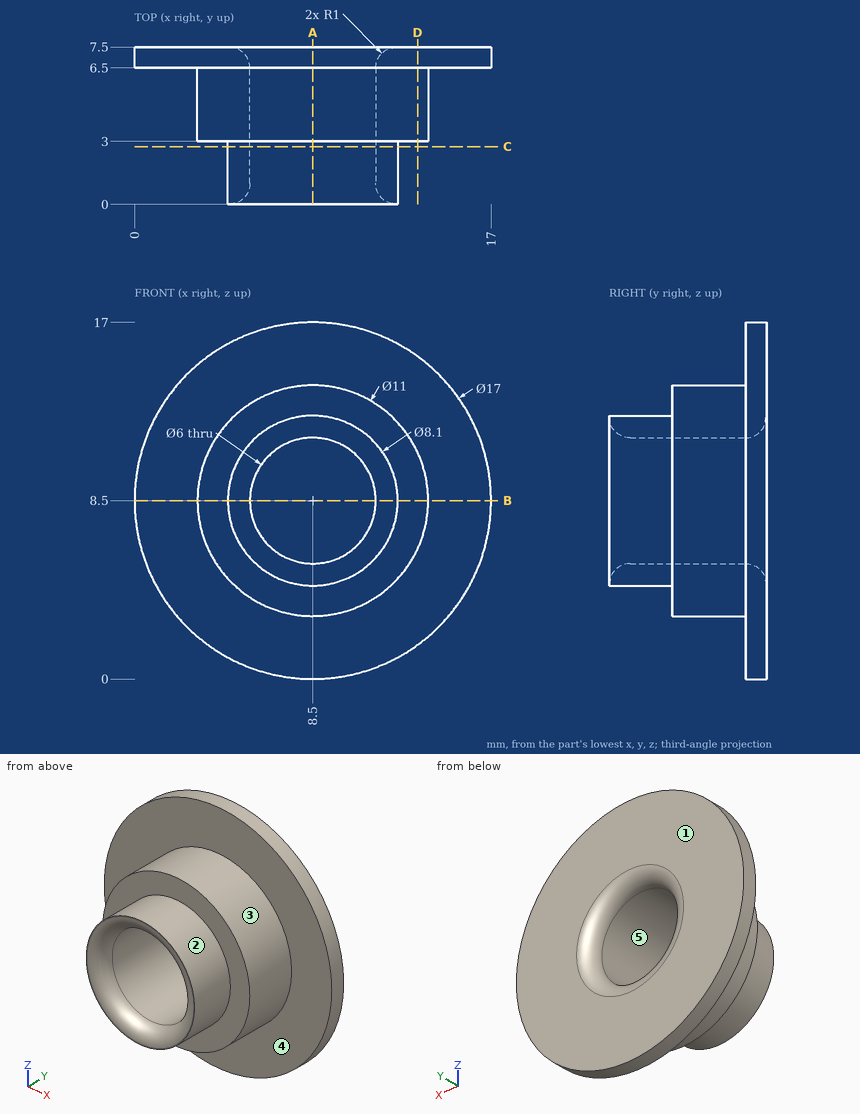
Geometry: see drawing. Coordinates: mm, zero at the bounding-box minimum. A direction names the side the tool comes from. Give positions to 0.01 mm unless a question says otherwise; leave off trailing zeros. Order: outer loops, then holes, each group sorted by start corner. A loop starts at its lowest first (then second) coordinate and runs counter-clockwise, first axis right, second up.
Q1. Section A-A on x = 8.5. Output: boundary loops of the cut face in (y, z).
Checked values:
outline: (0, 4.45) - (3, 4.45) - (3, 3) - (6.5, 3) - (6.5, 0) - (7.5, 0) - (7.5, 4.5) arc R1 ccw to (6.5, 5.5) - (1, 5.5) arc R1 ccw to (0, 4.5) - close; (0, 12.5) arc R1 ccw to (1, 11.5) - (6.5, 11.5) arc R1 ccw to (7.5, 12.5) - (7.5, 17) - (6.5, 17) - (6.5, 14) - (3, 14) - (3, 12.55) - (0, 12.55) - close
Q2. Ray query, probe 1 along Z at (x, y) = (8.5, 3.5); probe 2 along Y at (x, z) = (15.5, 8.25); probe 3 along X at (y, z) = (1, 6.25). Return the intervals inside material, ascending.
Checked values:
probe 1: z = 3 to 5.5, 11.5 to 14
probe 2: y = 6.5 to 7.5
probe 3: x = 5.13 to 6.52, 10.48 to 11.87
Q3. Section D-D on x = 13.5. Output: boundary loops of the cut face in (y, z).
Checked values:
outline: (3, 6.21) - (6.5, 6.21) - (6.5, 1.63) - (7.5, 1.63) - (7.5, 15.37) - (6.5, 15.37) - (6.5, 10.79) - (3, 10.79) - close
Q4. Section C-C on y = 2.75. Output: boundary loops of the cut face in (x, z).
Checked values:
outline: circle Ø8.1 at (8.5, 8.5); hole circle Ø6 at (8.5, 8.5)
Q5. Draft query along Z for the marked faces 3, 4 and 5. Return one class per face: +Z half, -Z half, draft (parallel to the pull), parting line (faces both ways), or undercut.
Checked values:
face 3: parting line
face 4: draft
face 5: undercut
Q6. Contact query for flat-ended pins moving along their axis: pin 1 Ø3 at (x, z) = (3.5, 3) entering from -Y; pin 2 Ø1 at (x, z) = (12, 4) entering from -Y. Output: stop coordinate, or through.
Checked values:
pin 1: stops at y = 6.5
pin 2: stops at y = 3
Q7. Set-up query: the marked faces 1 and 2. Return all of +Z, -Z, +X, -X, +Y, -Y with unobstructed straight access to the full face (end or side cutting, diameter ignored); none if empty.
Checked values:
face 1: +Z, -Z, +X, -X, +Y
face 2: -Y
Q8. Section B-B on z = 8.5. Output: boundary loops of the cut face in (x, y).
Checked values:
outline: (0, 6.5) - (3, 6.5) - (3, 3) - (4.45, 3) - (4.45, 0) - (4.5, 0) arc R1 ccw to (5.5, 1) - (5.5, 6.5) arc R1 ccw to (4.5, 7.5) - (0, 7.5) - close; (11.5, 1) arc R1 ccw to (12.5, 0) - (12.55, 0) - (12.55, 3) - (14, 3) - (14, 6.5) - (17, 6.5) - (17, 7.5) - (12.5, 7.5) arc R1 ccw to (11.5, 6.5) - close
